from build123d import *

# Parameters (mm, degrees)
F0_R     = 8.5
F1_DEPTH = 4
F2_R     = 5
F3_DEPTH = 100
F5_DEPTH = 3


with BuildPart() as f1:
    # F0 (on Top) → F1 (new body)
    with BuildSketch(Plane.XY):
        Circle(F0_R)
    extrude(amount=F1_DEPTH)

    # F2 (on Top) → F3 (join)
    with BuildSketch(Plane.XY):
        Circle(F2_R)
    extrude(amount=F3_DEPTH)

    # F4 (on face) → F5 (cut)
    with BuildSketch(Plane.XY.offset(100)):
        with BuildLine():
            Line((4.8989794856, 1), (1, 1))
            Line((1, 1), (1, -1))
            Line((1, -1), (4.8989794856, -1))
            ThreePointArc((4.8989794856, -1), (4.974680765, -0.50254481), (5, 0))
            ThreePointArc((5, 0), (4.974680765, 0.50254481), (4.8989794856, 1))
        make_face()
    extrude(amount=-F5_DEPTH, mode=Mode.SUBTRACT)


solid = f1.part
Geometry: final body of the model. Coordinates: model frame, mm. A direction names the side the tool comes from. Give positions to 0.01 mm unless a question says otherwise; leave off trailing zeros. Loops run counter-clockwise (first coordinate to the right, second up) from the corner with the lowest first, then second, coordinate; pieces in that order, holes last. Notation, with made-up numbers: M -8.75,27.5 L 13.25,27.5 A31 ccw 13.25,62.5 Z; hole C 84.5,0.5 d2. An arc over 180 degrees is marked long. Put each result on its own line as item: value. Start each with the question number.
1) Cut plane A-A (y = 0). Output: boundary loops of the cut face in (x, z), then the cut area to 3 significant figures.
2) Access query for faces 1 (the flat face through (3, 0, 97)), 2 (the cylindrical face through (4.57, 7.167, 1.972)). Directions: +Z, -Z, +X, -X, +Y, -Y. A direction counts if a zero-diameter tool reaches every point of the face in a straight line with its end or side. Return the directions, or none.
3) Ray query, line 1 along Z through (x, y) = (5.5, -4.5); line 2 along Y through (x, z) = (0, 86.5). Return the intervals inside material, ascending.
4) Contact query for flat-ended pins moving along their axis: pin 1 (3 mm diameter, centred on y = 1.5, z = 43.5, fed in from +X); pin 2 (3 mm diameter, centred on x = -2, y = 6.5, fed in from +Z); pin 3 (2.5 mm diameter, centred on x = 3.5, z = 98.5, fed in from +Y). Output: stop coordinate, or through.
5) Cut plane C-C (z = 88). Output: boundary loops of the cut face in (x, y), then the cut area to 3 significant figures.
6) Cut plane D-D (y = 4). Output: boundary loops of the cut face in (x, z), then the cut area to 3 significant figures.
7) Cut plane B-B (x = -3.75). Output: boundary loops of the cut face in (y, z).
8) Pull-direction query (Y, two-part tool) for faces 3 (the flat face through (3, 1, 99)), 4 (the cylindrical face through (-1.08, -4.88, 51.33)), 5 (the flat face through (4, -4, 4)); classes: pulls with the +Y half, pulls with the -Y half, needs draft (parallel to the pull), parting line crosses it, or undercut.
Verdict:
1. outline: M -8.5,0 L 8.5,0 L 8.5,4 L 5,4 L 5,97 L 1,97 L 1,100 L -5,100 L -5,4 L -8.5,4 Z
1. area: 1,020 mm2
2. face 1: +Z, +X
2. face 2: +Z, -Z
3. line 1: 0 to 4
3. line 2: -5 to 5
4. pin 1: x = 5
4. pin 2: z = 4
4. pin 3: y = 4.47
5. outline: C 0,0 d10
5. area: 78.5 mm2
6. outline: M -7.5,0 L 7.5,0 L 7.5,4 L 3,4 L 3,100 L -3,100 L -3,4 L -7.5,4 Z
6. area: 636 mm2
7. outline: M -7.63,0 L 7.63,0 L 7.63,4 L 3.31,4 L 3.31,100 L -3.31,100 L -3.31,4 L -7.63,4 Z
8. face 3: undercut
8. face 4: parting line crosses it
8. face 5: needs draft
